Could you check a few things on this drawing? It's one solid part, dimensions in mm from its lowest x, y, z. Give positions to 0.01 mm unless a question says otherwise; leave off trailing zeros. Write each loop counter-clockwise with the first axis right and the second up, starting at its lowest first coordinate (ties: lowest second). Pieces come first, ordered by that corner, then holes.
1. Suppose I cut it at B-B (y = 12.7). Please give me the cut outline in (x, z) (1 decimal).
2. Suppose I cut it at D-D (y = 18). Please give me the cut outline in (x, z), and give its area (3 significant figures).
3. I'm going to push flat-ended pins straight in: pin 1 (2 mm diameter, centred on y = 18.5, z = 0.5, fed in from -X); pin 2 (1.5 mm diameter, centred on y = 3, z = 4, fed in from -X). Where does each tip first touch, or does it pass through?
4. Suppose I cut it at A-A (z = 2.05). Give the number of separate pieces and of enclosed holes in the cut face, and give its area (3 significant figures).
5. Suppose I cut it at C-C (x = 8.5). Please give me the cut outline in (y, z) (1 decimal).
6. If I drill on probe 1 along Y at (x, z) = (8, 3.3); probe 2 along X at (y, z) = (14, 1.2) (1 decimal); probe 3 along X at (y, z) = (14.5, 2.5) (1 decimal), over which ranges is the centre line in solid material (lowest first)?
7. Thinking about a two-plate mould opening in X: for the marked faces 1, 2 and 3, which applies, pulls with the +X half, pulls with the -X half, needs draft (parallel to the pull), parting line crosses it, or undercut?
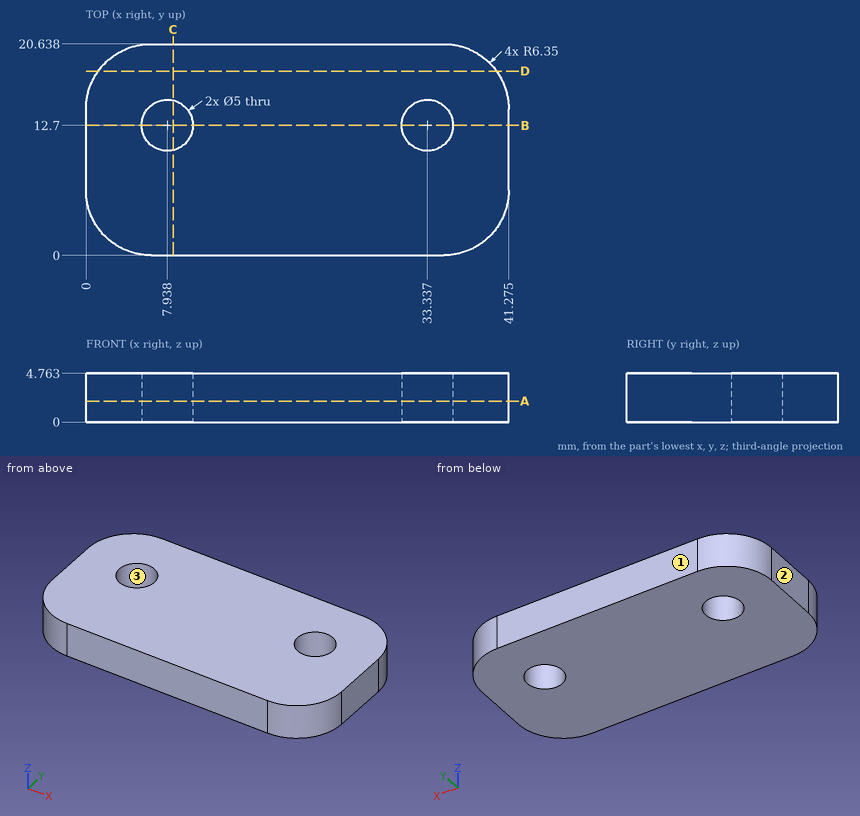
Checks:
1. outline: (0, 0) - (5.4, 0) - (5.4, 4.8) - (0, 4.8) - close; (10.4, 0) - (30.8, 0) - (30.8, 4.8) - (10.4, 4.8) - close; (35.8, 0) - (41.3, 0) - (41.3, 4.8) - (35.8, 4.8) - close
2. outline: (1.2, 0) - (40.08, 0) - (40.08, 4.76) - (1.2, 4.76) - close
2. area: 185 mm2
3. pin 1: stops at x = 0.87
3. pin 2: stops at x = 0.56
4. separate pieces: 1
4. enclosed holes: 2
4. area: 778 mm2
5. outline: (0, 0) - (10.3, 0) - (10.3, 4.8) - (0, 4.8) - close; (15.1, 0) - (20.6, 0) - (20.6, 4.8) - (15.1, 4.8) - close
6. probe 1: y = 0 to 10.2, 15.2 to 20.64
6. probe 2: x = 0 to 5.8, 10.1 to 31.2, 35.5 to 41.3
6. probe 3: x = 0 to 6.2, 9.7 to 31.6, 35.1 to 41.3
7. face 1: needs draft
7. face 2: pulls with the -X half
7. face 3: undercut
